Could you check a few things on this model? Use its own coordinates, in mm. Give positions to 0.01 mm unless a question says otherwise; leave off trailing zeros. Loops run counter-clockwise (first coordinate to the right, second up) from the corner with the lowest first, then second, coordinate; pieces in that order, holes last. Notation, with made-up numbers: M 57,-18 L 92,-18 A26 ccw 92,5 Z; hole C 80.5,81 d3. An arc over 180 degrees is marked long. Return JSON: item names as keys, results as strings. Group by question number.
1. If we section it at B-B (z = 0): Write out the boundary of the cut face in (x, y).
2. Please list where these lines run through material, in increasing order: line 1 (Z direction, x = 0.25, y = 1.8); line 2 (X direction, y = 1.9, z = 0.75); line 3 (X direction, y = 1.1, z = 2.5).
3. If we section it at A-A (x = 0): Write out the boundary of the cut face in (y, z).
4. If we section it at C-C (y = 0.5): Write out the boundary of the cut face in (x, z).
5. If we mould it in two halves opening along X, with no side actions, what happens to faces 1 (the flat face through (-14.5, 1, 0)), 2 (the cylindrical face through (-0.867, 0.986, -3.905)), 3 (the flat face through (14.5, 1, 0)), 4 (the flat face through (0, 1, -14.5))? For each: +X half, -X half, draft (parallel to the pull), parting line (faces both ways), or undercut.
Solid Edge part; units mm, degrees
sketch "Sketch1" plane through (0, 0, 0) normal (0, -1, 0) x (1, 0, 0)
  circle A0 centre (0, 0) radius 4
  line L0 (14.5, 14.5) -> (-14.5, 14.5)
  line L1 (-14.5, 14.5) -> (-14.5, -14.5)
  line L2 (-14.5, -14.5) -> (14.5, -14.5)
  line L3 (14.5, -14.5) -> (14.5, 14.5)
extrude "Protrusion1" add sketch "Sketch1" against normal blind 2
Answer:
{
 "1": {"outline": "M -14.5,0 L -4,0 L -4,2 L -14.5,2 Z; M 4,0 L 14.5,0 L 14.5,2 L 4,2 Z"},
 "2": {"line 1": "z = -14.5 to -3.99, 3.99 to 14.5", "line 2": "x = -14.5 to -3.93, 3.93 to 14.5", "line 3": "x = -14.5 to -3.12, 3.12 to 14.5"},
 "3": {"outline": "M 0,-14.5 L 2,-14.5 L 2,-4 L 0,-4 Z; M 0,4 L 2,4 L 2,14.5 L 0,14.5 Z"},
 "4": {"outline": "M -14.5,-14.5 L 14.5,-14.5 L 14.5,14.5 L -14.5,14.5 Z; hole C 0,0 d8"},
 "5": {"face 1": "-X half", "face 2": "undercut", "face 3": "+X half", "face 4": "draft"}
}
